Design review of the part built by this model. Coordinates are the model's own, in mm. A direction names the side the tool comes from. Round coordinates to 2 decimals unless told otherwise and drop trailing zeros. Write each loop counter-clockwise with the first axis right and the second up, starting at its lowest first coordinate (ties: lowest second). Pieces come first, ordered by that corner, then holes. Notation, with made-up numbers: (76.25, 10) -> (90.25, 10) arc R26 cw to (90.25, 36) -> close; hole circle Ø9 at (-14.75, 20.25). An arc over 180 degrees is marked (long way). Write item = value, one per line. Start each with the question number.
Item 1: Add section D-D, the plane z = 2.65. State how many separate pieces and enclosed holes the cut face has, then the cut area to 3 significant figures.
Item 2: Add section B-B, the plane x = 0. State the section outline as (y, z) points, then the cut area to 4 significant figures.
Item 3: Add section A-A, the plane y = 0. State the section outline as (x, z) points.
Item 4: Mouldability with a two-part tool opening along Y and no side actions: class faces 1 (the cylindrical face through (-0.176, -16.411, 2.465)), 2 (the flat face through (-16.22, 18.73, 2.46)), 3 (the cylindrical face through (20.976, -5.752, 2.465)) as released by +Y, released by -Y, zero draft, split by the parting line, or undercut.
Item 5: Machinability: for faces 4 (the cylindrical face through (0, 38, 2)), 5 (the cylindrical face through (8.21, -11.9, 2.54)), 6 (the flat face through (8.84, -14.67, 2.46)), which of the approach directions +Z, -Z, +X, -X, +Y, -Y give a long, thin tool a straight path to every point of the face, cutting with its end or side? Answer none if there is none.
Item 6: To check wall thickness, follow L1, parallel to Y at x = 0, z = 3.25; L2, parallel to Y at x = 1, z = 4.1; L3, parallel to X at y = 8, z = 4.2. State the ranges of each line that lie inside material, in increasing order.
Item 7: For pin 1 Ø2.5 at (x, y) = (0, -17.75) entering from +Z; pin 2 Ø2 at (x, z) = (-4, 4) entering from +Y, all flat-tipped, find the tip position at first contact; note any pin that passes through.
Item 8: Add section C-C, the plane x = -15. State the section outline as (y, z) points.
from build123d import *

# Parameters (mm, degrees)
SKETCH1_R           = 5
SKETCH1_R_2         = 1.35
BOSS_EXTRUDE1_DEPTH = 5
CONG_2_R            = 3


with BuildPart() as part:
    # Sketch1 → Boss-Extrude1 (new body)
    with BuildSketch(Plane.XY):
        with BuildLine():
            Line((7.433976594, -11.567129808), (10.756607468, -18.903912182))
            ThreePointArc((10.756607468, -18.903912182), (20.44660049, -7.416132981), (20.37430597, 7.6125))
            Line((20.37430597, 7.6125), (12.177746097, 29.55))
            ThreePointArc((12.177746097, 29.55), (0, 38), (-12.177746097, 29.55))
            Line((-12.177746097, 29.55), (-20.37430597, 7.6125))
            ThreePointArc((-20.37430597, 7.6125), (-15.56616527, -15.190687897), (7.112849411, -20.554071939))
            Line((7.112849411, -20.554071939), (3.790218537, -13.217289565))
            ThreePointArc((3.790218537, -13.217289565), (-5.672424163, 12.525418321), (7.433976594, -11.567129808))
        make_face()
        with Locations((0, 25)):
            Circle(SKETCH1_R, mode=Mode.SUBTRACT)
        with Locations((0, -17.75)):
            Circle(SKETCH1_R_2, mode=Mode.SUBTRACT)
        with Locations((15.371950917, 8.875)):
            Circle(SKETCH1_R_2, mode=Mode.SUBTRACT)
        with Locations((-15.371950917, 8.875)):
            Circle(SKETCH1_R_2, mode=Mode.SUBTRACT)
    extrude(amount=BOSS_EXTRUDE1_DEPTH)

    # Congé2
    cong_2_edges = [part.edges().sort_by_distance(p)[0] for p in [
        (3.790218537, -13.217289565, 2.5),
        (7.112849411, -20.554071939, 2.5),
        (10.756607468, -18.903912182, 2.5),
        (7.433976594, -11.567129808, 2.5),
    ]]
    fillet(cong_2_edges, radius=CONG_2_R)


solid = part.part
Result set:
q1.separate_pieces = 1
q1.enclosed_holes = 4
q1.area = 1,200 mm²
q2.outline = (-21.75, 0) -> (-19.1, 0) -> (-19.1, 5) -> (-21.75, 5) -> close; (-16.4, 0) -> (-13.75, 0) -> (-13.75, 5) -> (-16.4, 5) -> close; (13.75, 0) -> (20, 0) -> (20, 5) -> (13.75, 5) -> close; (30, 0) -> (38, 0) -> (38, 5) -> (30, 5) -> close
q2.area = 97.75 mm²
q3.outline = (-21.75, 0) -> (-13.75, 0) -> (-13.75, 5) -> (-21.75, 5) -> close; (13.75, 0) -> (21.75, 0) -> (21.75, 5) -> (13.75, 5) -> close
q4.face_1 = undercut
q4.face_2 = released by +Y
q4.face_3 = split by the parting line
q5.face_4 = +Z, -Z, +Y
q5.face_5 = +Z, -Z
q5.face_6 = +Z, -Z, -Y
q6.L1 = -21.75 to -19.1, -16.4 to -13.75, 13.75 to 20, 30 to 38
q6.L2 = -21.73 to -18.66, -16.84 to -13.71, 13.71 to 20.1, 29.9 to 37.96
q6.L3 = -20.23 to -16.4, -14.34 to -11.18, 11.18 to 14.34, 16.4 to 20.23
q7.pin_1 = through
q7.pin_2 = 37.65
q8.outline = (-15.75, 0) -> (7.58, 0) -> (7.58, 5) -> (-15.75, 5) -> close; (10.17, 0) -> (22, 0) -> (22, 5) -> (10.17, 5) -> close
